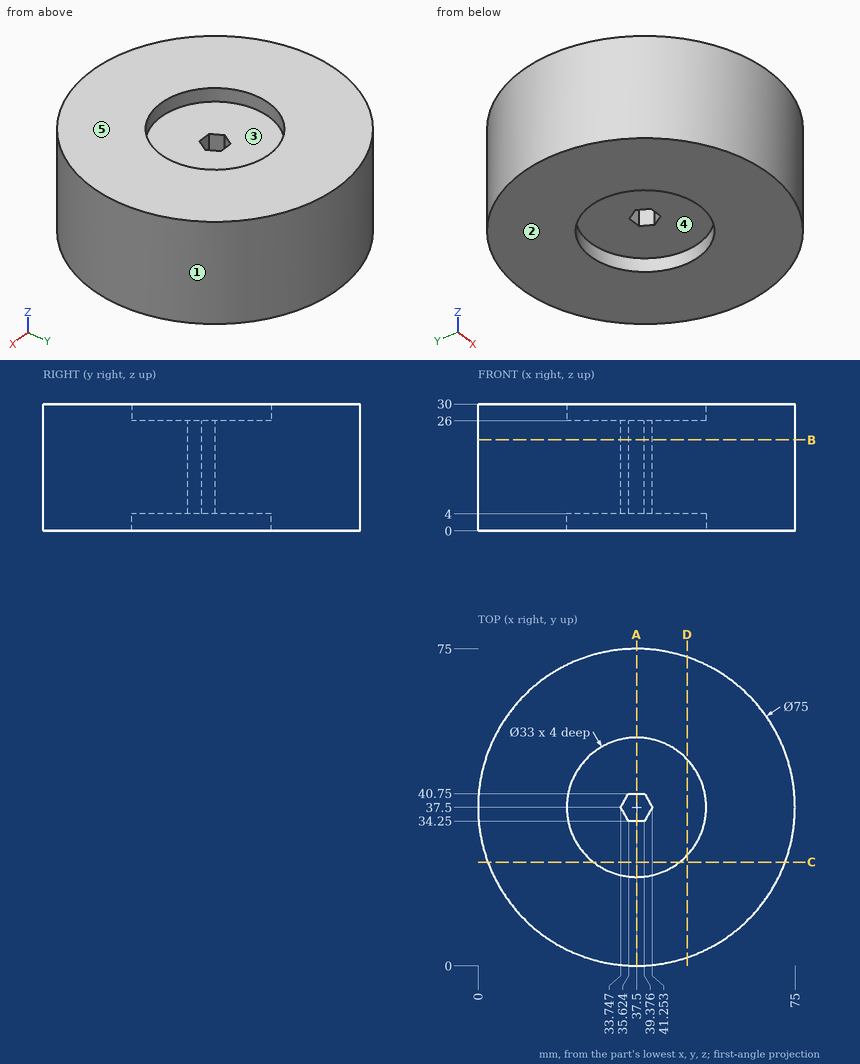
Job drawing, mm, ordinate dimensions from the low corner. One solid piece. A direction names the side the tool comes from. Coordinates: 2 decimals unless noted, no trailing zeros. Order: outer loops, then holes, each group sorted by start corner. A loop starts at its lowest first (then second) coordinate and runs counter-clockwise, first axis right, second up. Notation, with made-up numbers: (73, 46) -> (123, 46) arc R26 ccw to (123, 73) -> close; hole circle Ø5 at (24, 29.5). An arc over 180 degrees is marked (long way). Return JSON: item names as keys, results as strings. Group by question number.
Item 1: Pull direction X, two halves, no side cores. Call the marked faces 1, 2 and 3: pulls with the +X half, pulls with the -X half, needs draft (parallel to the pull), parting line crosses it, or undercut.
Item 2: Saw through at B-B on z = 21.5. Write the cut outline in (x, y), then the cut area to 3 significant figures.
Item 3: Tool access for the marked faces 4 and 5: list every direction of +Z, -Z, +X, -X, +Y, -Y with a clear straight run to the whole face (end or side of a thin tool).
Item 4: Saw through at A-A on x = 37.5. Write the cut outline in (y, z).
Item 5: Flat gauge pins, fed straight in: P1, Ø10, axis at x = 41, y = 41, coming from the +Z side; P2, Ø3, axis at y = 40.5, z = 23, coming from the -X side; P3, Ø12, axis at y = 30, z = 20.5, coming from the +X side. Where does each tip first touch, or does it go through?
Item 6: Wall check: line 1 along Y through (x, z) = (37.5, 28.9); line 2 along X through (y, z) = (35, 27); line 3 along X through (y, z) = (47.5, 2.25) (1 decimal). Give the ranges that are in metal, low to high. Write a range as [from, to].
Item 7: Saw through at C-C on y = 24.5. Write the cut outline in (x, z) (1 decimal).
Item 8: Saw through at D-D on x = 49.5. Write the cut outline in (y, z) (1 decimal).
Values found:
{
 "1": {"face 1": "parting line crosses it", "face 2": "needs draft", "face 3": "undercut"},
 "2": {"outline": "circle Ø75 at (37.5, 37.5); hole (33.75, 37.5) -> (35.62, 34.25) -> (39.38, 34.25) -> (41.25, 37.5) -> (39.38, 40.75) -> (35.62, 40.75) -> close", "area": "4,380 mm2"},
 "3": {"face 4": "-Z", "face 5": "+Z, +X, -X, +Y, -Y"},
 "4": {"outline": "(0, 0) -> (21, 0) -> (21, 4) -> (34.25, 4) -> (34.25, 26) -> (21, 26) -> (21, 30) -> (0, 30) -> close; (40.75, 4) -> (54, 4) -> (54, 0) -> (75, 0) -> (75, 30) -> (54, 30) -> (54, 26) -> (40.75, 26) -> close"},
 "5": {"P1": "stops at z = 26", "P2": "stops at x = 0.03", "P3": "stops at x = 74.97"},
 "6": {"line 1": "y = [0, 21], [54, 75]", "line 2": "x = [0.08, 21.19], [53.81, 74.92]", "line 3": "x = [1.4, 24.4], [50.6, 73.6]"},
 "7": {"outline": "(2.3, 0) -> (27.3, 0) -> (27.3, 4) -> (47.7, 4) -> (47.7, 0) -> (72.7, 0) -> (72.7, 30) -> (47.7, 30) -> (47.7, 26) -> (27.3, 26) -> (27.3, 30) -> (2.3, 30) -> close"},
 "8": {"outline": "(2, 0) -> (26.2, 0) -> (26.2, 4) -> (48.8, 4) -> (48.8, 0) -> (73, 0) -> (73, 30) -> (48.8, 30) -> (48.8, 26) -> (26.2, 26) -> (26.2, 30) -> (2, 30) -> close"}
}
